Geometry check sheet. Reference: the model listing, model coordinates, mm. A direction names the side the tool comes from. Coordinates: 2 decimals unless noted, no trailing zeros. Write each loop counter-clockwise with the first axis right and the second up, starting at its lowest first coordinate (ties: lowest second). Pieces come first, ordered by that corner, then holes. Notation, with made-up numbers: (21.25, 46.5) -> (41.25, 46.5) arc R33 ccw to (41.25, 76.5) -> close; hole circle Ø10 at (1.25, -19.5). An arc over 180 degrees is marked (long way). Answer in a Markdown table with one row per item. Add a question column.
Q1. Section check B-B, the plane y = 131.5. Record the boundary of the cut face in (x, z).
Q2. Release check for a two-part mould opening along Y. For faces 1 (the face through (-1, 99, 40)), 2 (the face through (76, 200, 30)), 3 (the face through (-1, 0, -1)) record: pulls with the +Y half, pulls with the -Y half, needs draft (parallel to the pull), parting line crosses it, or undercut.
Q3. Thickness scan on line 1 (Z direction, x = 72.5, y = 177); line 2 (Y direction, x = -45.5, z = 114); line 3 (Y direction, x = 122, z = -135.5). Record the ranges inside material, lowest first.
Q4. Gauge pin test, flat end, axial feed: P1, Ø4, axis at x = -50, y = 130, coming from the -Z side. Record the tip position at first contact, or that the pin passes through.
Q5. Tool access check on faces 4 (the face through (80, 99, 1)), 5 (the face through (1, 200, -56)), 6 (the face through (-80, 99, 1)). Record the directions out of +Z, -Z, +X, -X, +Y, -Y that give a thin tool (end or side, any length) a straight path to the whole face; none if there is none.
Q6. Section check A-A, the plane x = 0. Record the boundary of the cut face in (y, z), and give its area (3 significant figures).
```python
from build123d import *

# Parameters (mm, degrees)
SKETCH_1_W      = 160
SKETCH_1_H      = 80
EXTRUDE_1_DEPTH = 200


with BuildPart() as part:
    # 草图1 → 凸台-拉伸1 (new body)
    with BuildSketch(Plane(origin=(0, 0, 0), x_dir=(1, 0, 0), z_dir=(0, 1, 0))):
        Rectangle(SKETCH_1_W, SKETCH_1_H)
    extrude(amount=EXTRUDE_1_DEPTH)

    # 草图2 → 旋转1 (revolve)
    with BuildSketch(Plane.XY):
        Polygon((0, 230), (-200, 230), (-80, 200), (0, 200), align=None)
    revolve(axis=Axis((0, 242.596859874, 0), (0, -1, 0)))


solid = part.part
```
Calculated:
| question | item | result |
|---|---|---|
| 1 | outline | (-80, -40) -> (80, -40) -> (80, 40) -> (-80, 40) -> close |
| 2 | face 1 | needs draft |
| 2 | face 2 | undercut |
| 2 | face 3 | pulls with the -Y half |
| 3 | line 1 | z = -40 to 40 |
| 3 | line 2 | y = 210.69 to 230 |
| 3 | line 3 | y = 225.58 to 230 |
| 4 | P1 | stops at z = -40 |
| 5 | face 4 | +Z, -Z, +X, -Y |
| 5 | face 5 | -Z, +X, -X, -Y |
| 5 | face 6 | +Z, -Z, -X, -Y |
| 6 | outline | (0, -40) -> (200, -40) -> (200, -80) -> (230, -200) -> (230, 200) -> (200, 80) -> (200, 40) -> (0, 40) -> close |
| 6 | area | 24,400 mm² |
